Here's how the part is built. I have some questions about the finished solid (model axes, mm). A direction names the side the tool comes from. Round coordinates to 2 decimals unless told otherwise and drop trailing zeros. Order: outer loops, then holes, each group sorted by start corner. A loop starts at its lowest first (then second) coordinate and runs counter-clockwise, first axis right, second up. Notation, with made-up numbers: (-5.75, 49) - (17.25, 49) arc R5 ccw to (17.25, 54) - close; hole circle Ø3 at (-25.75, -24.5). An arc over 180 degrees is marked (long way). Answer as a JSON object with one key per item and string values.
```python
from build123d import *

# Parameters (mm, degrees)
SKETCH_W        = 110
SKETCH_H        = 110
PAD_DEPTH       = 6
POCKET_DEPTH    = 110
POCKET001_DEPTH = 110
SKETCH003_W     = 80
SKETCH003_H     = 80
POCKET002_DEPTH = 6


with BuildPart() as part:
    # Sketch → Pad (new body)
    with BuildSketch(Plane.XY):
        Rectangle(SKETCH_W, SKETCH_H)
    extrude(amount=PAD_DEPTH)

    # Sketch002 (on Face3 of Pad) → Pocket (cut)
    with BuildSketch(Plane.XZ.offset(55)):
        Polygon((55, 6), (55, 0), (49, 0), align=None)
        Polygon((-55, 6), (-55, 0), (-49, 0), align=None)
    extrude(amount=-POCKET_DEPTH, mode=Mode.SUBTRACT)

    # Sketch001 (on Face2 of Pad) → Pocket001 (cut)
    with BuildSketch(Plane.YZ.offset(55)):
        Polygon((55, 6), (55, 0), (49, 0), align=None)
        Polygon((-55, 6), (-55, 0), (-49, 0), align=None)
    extrude(amount=-POCKET001_DEPTH, mode=Mode.SUBTRACT)

    # Sketch003 (on Face1 of Pocket001) → Pocket002 (cut)
    with BuildSketch(Plane.XY.offset(6)):
        Rectangle(SKETCH003_W, SKETCH003_H)
    extrude(amount=-POCKET002_DEPTH, mode=Mode.SUBTRACT)


solid = part.part
```
1. For P1, Ø2, axis at y = -15, z = 2, coming from the -X side; P2, Ø1.8, axis at y = 14.5, z = 4.5, coming from the +X side; P3, Ø3, axis at x = 40, y = 38, coming from the -Z side; P4, Ø1.8, axis at y = 5.5, z = 2, coming from the -X side, each with a flat end and sliding along its axis, tell me the tip position at first contact or that it passes through.
Responses:
{"P1": "x = -52", "P2": "x = 54.4", "P3": "z = 0", "P4": "x = -51.9"}
2. Imagine slicing it at A-A (x = 9). List the corners of the cut face in (y, z) for me, plus the area to 3 significant figures.
Responses:
{"outline": "(-55, 6) - (-49, 0) - (-40, 0) - (-40, 6) - close; (40, 0) - (49, 0) - (55, 6) - (40, 6) - close", "area": "144 mm2"}
3. If I drill on L1, parallel to X at y = 0, z = 1.5; L2, parallel to Y at x = -26, z = 1.75; L3, parallel to X at y = -21, z = 5.25, over which ranges is the centre line in solid material (lowest first)? Write a range as [from, to].
Responses:
{"L1": "[-50.5, -40], [40, 50.5]", "L2": "[-50.75, -40], [40, 50.75]", "L3": "[-54.25, -40], [40, 54.25]"}
4. Imagine slicing it at D-D (x = 43.5). List the corners of the cut face in (y, z) for me, plus the area to 3 significant figures.
Responses:
{"outline": "(-55, 6) - (-49, 0) - (49, 0) - (55, 6) - close", "area": "624 mm2"}
5. Imagine slicing it at C-C (z = 3.25). List the corners of the cut face in (x, y) for me.
Responses:
{"outline": "(-52.25, -52.25) - (52.25, -52.25) - (52.25, 52.25) - (-52.25, 52.25) - close; hole (-40, -40) - (40, -40) - (40, 40) - (-40, 40) - close"}
6. Thinking about a two-plate mould opening in Y: for faces 1 (the face through (43, 1, 0)), 2 (the face through (-1, -40, 3)), 3 (the face through (1, -52, 3)), which applies, pulls with the +Y half, pulls with the -Y half, needs draft (parallel to the pull), parting line crosses it, or undercut?
Responses:
{"face 1": "needs draft", "face 2": "undercut", "face 3": "pulls with the -Y half"}
7. For faces 4 (the face through (52, -1, 3)), 5 (the face through (40, -1, 3)), which set-ups out of +Z, -Z, +X, -X, +Y, -Y let a thin tool reach every point of the face, with its end or its side?
Responses:
{"face 4": "-Z, +X, +Y, -Y", "face 5": "+Z, -Z"}
